Model file for the job. Use its own axes, mm. Face numbers are marked on the shaded views. A direction names the side the tool comes from. Give positions to 0.01 mm unless a question says otherwise; leave off trailing zeros. Loops run counter-clockwise (first coordinate to the right, second up) from the corner with the lowest first, then second, coordinate; pieces in that order, holes last. Notation, with made-up numbers: (20, -18) -> (64, -18) arc R8 cw to (64, -14) -> close; hole circle Ø5 at (5.5, -38). An arc over 180 degrees is marked (long way). Use CSV: the item, a comma, the result in double quotes. Start each with the question number.
(1) 3-axis set-ups, long thin cutter, end or side, ignore diameter. For the marked faces 5 and 6: which of +Z, -Z, +X, -X, +Y, -Y reach the whole face in a straight line?
(2) Cut at A-A on x = 4. Write the cut outline in (y, z), then the cut area to 3 significant figures.
(3) Cut at C-C on y = 1.05. Write the cut outline in (x, z).
(4) Pull direction Z, two halves, no side cores. Call the marked faces 1, 2, 3 and 4: pulls with the +Z half, pulls with the -Z half, needs draft (parallel to the pull), parting line crosses it, or undercut.
(5) Flat gauge pins, fed straight in: pin 1 (4 mm diameter, centred on x = 4, z = -3.75, fed in from -Y); pin 2 (1.5 mm diameter, centred on x = 7, z = -6.5, fed in from -Y); pin 3 (3 mm diameter, centred on x = 4, z = -4, fed in from -Y). Where does each tip first touch, or does it go through?
(6) Cut at B-B on z = -3.75. Write the cut outline in (x, y), then the cut area to 3 significant figures.
(7) Cut at D-D on x = 2. Write the cut outline in (y, z).
(8) Drill centre lines: probe 1 along Z at (x, y) = (4.25, -0.2); probe 2 along Y at (x, z) = (2.25, -2.5); probe 3 along X at (y, z) = (0.6, -5.25). Where is each one in solid material? Low to high.
from build123d import *

# Parameters (mm, degrees)
SKETCH1_W               = 8
SKETCH1_H               = 8
BOSS_EXTRUDE1_DEPTH     = 3
CUT_EXTRUDE1_DEPTH      = 12.704699911
CUT_EXTRUDE1_DEPTH_BACK = 12.704699911
CUT_EXTRUDE2_DEPTH      = 11
SKETCH4_R               = 1.8
CUT_EXTRUDE3_DEPTH      = 0.8
SKETCH5_W               = 8
SKETCH5_H               = 1
BOSS_EXTRUDE2_DEPTH     = 2
FILLET1_R               = 4
CUT_EXTRUDE4_DEPTH      = 0.4


with BuildPart() as part:
    # Sketch1 → Boss-Extrude1 (new body)
    with BuildSketch(Plane(origin=(0, 0, 0), x_dir=(1, 0, 0), z_dir=(0, 1, 0))):
        with Locations((4, 4)):
            Rectangle(SKETCH1_W, SKETCH1_H)
    extrude(amount=BOSS_EXTRUDE1_DEPTH)

    # Sketch2 → Cut-Extrude1 (cut, two sides: drawn at the far end of the back side and taken through both)
    with BuildSketch(Plane.XY.offset(-CUT_EXTRUDE1_DEPTH_BACK)):
        Polygon((0, 0), (0.6, 3), (0, 3), align=None)
        Polygon((8, 0), (7.4, 3), (8, 3), align=None)
    extrude(amount=CUT_EXTRUDE1_DEPTH + CUT_EXTRUDE1_DEPTH_BACK, mode=Mode.SUBTRACT)

    # Sketch3 → Cut-Extrude2 (cut)
    with BuildSketch(Plane(origin=(0, 0, 0), x_dir=(0, 0, -1), z_dir=(1, 0, 0))):
        Polygon((0, 0), (0.6, 3), (0, 3), align=None)
        Polygon((8, 3), (7.4, 3), (8, 0), align=None)
    extrude(amount=CUT_EXTRUDE2_DEPTH, mode=Mode.SUBTRACT)

    # Sketch4 → Cut-Extrude3 (cut)
    with BuildSketch(Plane.XZ):
        with Locations(Location((4, -3.75, 0), (0, 0, 270))):
            Circle(SKETCH4_R)
    extrude(amount=-CUT_EXTRUDE3_DEPTH, mode=Mode.SUBTRACT)

    # Sketch5 → Boss-Extrude2 (add)
    with BuildSketch(Plane.XZ):
        with Locations((4, -7.5)):
            Rectangle(SKETCH5_W, SKETCH5_H)
    extrude(amount=BOSS_EXTRUDE2_DEPTH)

    # Fillet1
    # the kernel refuses this fillet: 4 mm, written as the material it takes off along each edge
    with BuildSketch(Plane(origin=(8, -2, -16.660254038), x_dir=(0, 1, 0), z_dir=(0, 0, 1)), Plane(origin=(0, -2, 1.660254038), x_dir=(0, 1, 0), z_dir=(0, 0, -1))) as fillet1_piece_1:
        with BuildLine():
            CenterArc((4, 3.464101615), FILLET1_R, 180, 60)
            Line((0, 3.464101615), (-0.08, 3.464101615))
            Line((-0.08, 3.464101615), (-0.08, 0))
            Line((-0.08, 0), (0, -0.08))
            ThreePointArc((0, -0.08), (1, -0.08), (1.96, -0.069282032))
            Line((1.96, -0.069282032), (2, 0))
        make_face()
    extrude(amount=18.320508076, mode=Mode.SUBTRACT)

    # Sketch6 → Cut-Extrude4 (cut)
    with BuildSketch(Plane(origin=(0, 3, 0), x_dir=(1, 0, 0), z_dir=(0, 1, 0))):
        Polygon((3.652362984, 2.002856352), (3.652362984, 5.336189685), (2.472875805, 5.336189685), (2.472875805, 6.002856352), (5.601080933, 6.002856352), (5.601080933, 5.336189685), (4.421593754, 5.336189685), (4.421593754, 2.002856352), align=None)
    extrude(amount=-CUT_EXTRUDE4_DEPTH, mode=Mode.SUBTRACT)


solid = part.part
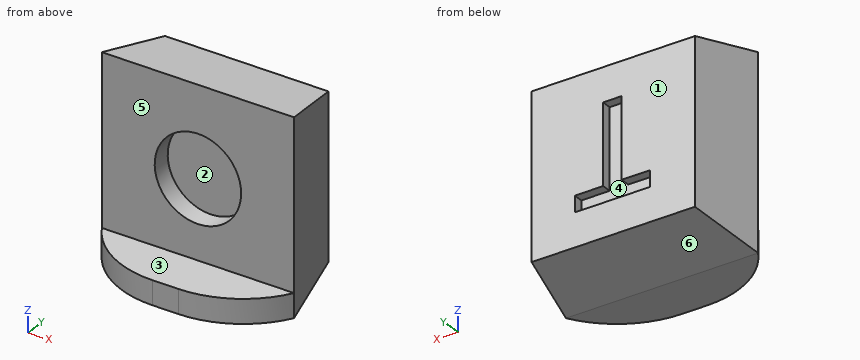
Check result:
1,face 5,"+Z, +X, -X, -Y"
1,face 6,"-Z, +X, -X, +Y"
2,outline,"(-2, -8) -> (0, -8) -> (3, -7.4) -> (3, -6) -> (2.6, -6) -> (2.6, -2) -> (3, -2) -> (3, -0.6) -> (0, 0) -> (0, -1.95) -> (0.8, -1.95) -> (0.8, -5.55) -> (0, -5.55) -> (0, -7) -> (-2, -7) -> close"
2,area,"19.7 mm²"
3,outline,"(0.21, -7.79) -> (7.79, -7.79) -> (7.79, -0.21) -> (0.21, -0.21) -> close"
4,face 1,"needs draft"
4,face 2,"undercut"
4,face 3,"pulls with the +Z half"
4,face 4,"undercut"
5,pin 1,"y = 0"
5,pin 2,"y = -1.52"
5,pin 3,"y = 0.8"
6,outline,"(0, 0) -> (2.2, 0) -> (2.2, 0.8) -> (5.8, 0.8) -> (5.8, 0) -> (8, 0) -> (7.4, 3) -> (4.42, 3) -> (4.42, 2.6) -> (3.65, 2.6) -> (3.65, 3) -> (0.6, 3) -> close"
6,area,"19.0 mm²"
7,outline,"(-1.72, -8) -> (0, -8) -> (3, -7.4) -> (3, -0.6) -> (0, 0) -> (0, -7) -> (-1.72, -7) -> close"
8,probe 1,"-8 to -7"
8,probe 2,"0 to 3"
8,probe 3,"0.12 to 3.01, 4.99 to 7.88"
